from build123d import *

# Parameters (mm, degrees)
SKETCH_R        = 1.75
PAD_DEPTH       = 2
PAD001_DEPTH    = 2
SKETCH002_R     = 3.25
PAD002_DEPTH    = 7
SKETCH003_R     = 6
SKETCH003_R_2   = 3
PAD003_DEPTH    = 11
CHAMFER_SIZE    = 2
CHAMFER001_SIZE = 0.75


with BuildPart() as part:
    # Sketch → Pad (new body)
    with BuildSketch(Plane.XY):
        with BuildLine():
            Line((-15.146068, 15.146068), (-9.146068, 15.146068))
            Line((-9.146068, 15.146068), (4.996068, 1.003932))
            Line((4.996068, 1.003932), (4.996068, -4.996068))
            Line((4.996068, -4.996068), (-15.146068, -4.996068))
            Line((-15.146068, -4.996068), (-122.792176, -116.931614))
            ThreePointArc((-137.207846, -103.068409), (-136.931603, -117.207835), (-122.792176, -116.931614))
            Line((-23.52342, 15.146068), (-137.207846, -103.068409))
            Line((-15.146068, 15.146068), (-23.52342, 15.146068))
        make_face()
        Circle(SKETCH_R, mode=Mode.SUBTRACT)
        with Locations((-10.15, 10.15)):
            Circle(SKETCH_R, mode=Mode.SUBTRACT)
    extrude(amount=-PAD_DEPTH)

    # Sketch001 → Pad001 (join)
    with BuildSketch(Plane.XY):
        Polygon((-9.146068, 15.146068), (-15.146068, 15.146068), (-15.146068, 9.146068), (-1.003932, -4.996068), (4.996068, -4.996068), (4.996068, 1.003932), align=None)
        Polygon((-0.841162, -3.139259), (2.298097, -2.298097), (3.139259, 0.841162), (0.841162, 3.139259), (-2.298097, 2.298097), (-3.139259, -0.841162), align=None, mode=Mode.SUBTRACT)
        Polygon((-7.851903, 7.851903), (-7.010741, 10.991162), (-9.308838, 13.289259), (-12.448097, 12.448097), (-13.289259, 9.308838), (-10.991162, 7.010741), align=None, mode=Mode.SUBTRACT)
    extrude(amount=PAD001_DEPTH)

    # Sketch002 → Pad002 (join)
    with BuildSketch(Plane.XY):
        with Locations((-130, -110)):
            Circle(SKETCH002_R)
    extrude(amount=PAD002_DEPTH)

    # Sketch003 → Pad003 (join)
    with BuildSketch(Plane.XY):
        with Locations((-130, -110)):
            Circle(SKETCH003_R)
        with Locations((-130, -110)):
            Circle(SKETCH003_R_2, mode=Mode.SUBTRACT)
    extrude(amount=PAD003_DEPTH)

    # Chamfer
    chamfer_edges = [part.edges().sort_by_distance(p)[0] for p in [
        (-15.146068, -4.996068, -1),
        (-23.52342, 15.146068, -1),
    ]]
    chamfer(chamfer_edges, length=CHAMFER_SIZE)

    # Chamfer001
    chamfer001_edges = [part.edges().sort_by_distance(p)[0] for p in [
        (-133, -110, 11),
        (-136, -110, 0),
        (-8.075, 2.075, 0),
        (-15.146068, 12.146068, 0),
    ]]
    chamfer(chamfer001_edges, length=CHAMFER001_SIZE)


solid = part.part
Could you check a few things on this model? Use its own coordinates, in mm. A direction names the side the tool comes from. Give positions to 0.01 mm unless a question says otherwise; leave off trailing zeros. Loops run counter-clockwise (first coordinate to the right, second up) from the corner with the lowest first, then second, coordinate; pieces in that order, holes last. Notation, with made-up numbers: (43, 62.5) -> (73, 62.5) arc R24 cw to (73, 82.5) -> close; hole circle Ø9 at (-10, 24). An arc over 180 degrees is marked (long way). Answer as CSV lines item,"result". Start each with the question number.
(1) If we section it at C-C on y = -81.5: Write out the boundary of the cut face in (x, z).
(2) If we section it at D-D on x = -60: Write out the boundary of the cut face in (y, z).
(3) If we section it at A-A on y = -110: Write out the boundary of the cut face in (x, z).
(4) I need wall thicknesses on probe 1 along Y at (x, z) = (-10.15, -0.35); probe 2 along Y at (x, z) = (-130, 9.4); probe 3 along Z at (x, y) = (-83, -69.5). Which ranges of each line are inside material? Lowest first, please.
(5) Which directions (+Z, -Z, +X, -X, +Y, -Y) give clear straight access to the entire face, cutting with the end or side of a thin tool? Please do faces 1 (the cylindrical face through (-127.14, -109.1, 8.6)), 2 (the flat face through (-14, 15.146, 0)), 3 (the flat face through (-8, 2, 1)).
(6) I'm going to push flat-ended pins straight in: pin 1 Ø1.9 at (x, y) = (-9.5, 10) entering from +Z; pin 2 Ø12 at (x, y) = (-33.5, -24.5) entering from +Z; pin 3 Ø6.5 at (x, y) = (-129, -110) entering from +Z; pin 4 Ø3 at (y, z) = (-61.5, 0.5) entering from -X. Where does each tip first touch, or does it pass through?
(7) We'd pull the mould along X, two halves only. Please class faces 4 (the flat face through (-130, -110, 7)), 5 (the flat face through (4.996, -2, 0)), 6 (the flat face through (-12, 9, 0)), 7 (the flat face through (-127, -107, 11)): released by +X, released by -X, zero draft, split by the parting line, or undercut.
(8) If we section it at B-B on x = -130: Write out the boundary of the cut face in (y, z), then the cut area to 3 significant figures.
Computed:
1,outline,"(-116.47, -2) -> (-88.72, -2) -> (-88.72, 0) -> (-116.47, 0) -> close"
2,outline,"(-51.64, -2) -> (-22.78, -2) -> (-22.78, 0) -> (-51.64, 0) -> close"
3,outline,"(-140, -2) -> (-116.13, -2) -> (-116.13, 0) -> (-123.25, 0) -> (-124, 0.75) -> (-124, 11) -> (-126.25, 11) -> (-127, 10.25) -> (-127, 7) -> (-133, 7) -> (-133, 10.25) -> (-133.75, 11) -> (-136, 11) -> (-136, 0.75) -> (-136.75, 0) -> (-140, 0) -> close"
4,probe 1,"y = -5 to 8.4, 11.9 to 15.15"
4,probe 2,"y = -116 to -113, -107 to -104"
4,probe 3,"z = -2 to 0"
5,face 1,"+Z"
5,face 2,"+Z, -Z, +X, -X, +Y"
5,face 3,"+Z, -X, -Y"
6,pin 1,"passes through"
6,pin 2,"stops at z = 0"
6,pin 3,"stops at z = 11"
6,pin 4,"stops at x = -98.59"
7,face 4,"undercut"
7,face 5,"released by +X"
7,face 6,"undercut"
7,face 7,"zero draft"
8,outline,"(-120, -2) -> (-95.57, -2) -> (-95.57, 0) -> (-103.25, 0) -> (-104, 0.75) -> (-104, 11) -> (-106.25, 11) -> (-107, 10.25) -> (-107, 7) -> (-113, 7) -> (-113, 10.25) -> (-113.75, 11) -> (-116, 11) -> (-116, 0.75) -> (-116.75, 0) -> (-120, 0) -> close"
8,area,"157 mm2"
